from build123d import *

# Parameters (mm, degrees)
SKETCH1_R           = 3.25
SKETCH1_R_2         = 1.75
BOSS_EXTRUDE1_DEPTH = 10


with BuildPart() as part:
    # Sketch1 → Boss-Extrude1 (new body)
    with BuildSketch(Plane.XY):
        with BuildLine():
            Line((75.75, 8.25), (0, 8.25))
            ThreePointArc((0, 8.25), (-8.25, 0), (0, -8.25))
            Line((0, -8.25), (64.25, -8.25))
            Line((64.25, -8.25), (64.25, -19))
            ThreePointArc((64.25, -19), (70, -24.75), (75.75, -19))
            Line((75.75, -19), (75.75, 8.25))
        make_face()
        Circle(SKETCH1_R, mode=Mode.SUBTRACT)
        with Locations((70, -11)):
            Circle(SKETCH1_R_2, mode=Mode.SUBTRACT)
        with Locations((70, -19)):
            Circle(SKETCH1_R_2, mode=Mode.SUBTRACT)
    extrude(amount=BOSS_EXTRUDE1_DEPTH)


solid = part.part
The model under review builds one solid part; all positions refer to its coordinate system, in mm. A direction names the side the tool comes from. Give positions to 0.01 mm unless a question says otherwise; leave off trailing zeros. Write each loop counter-clockwise with the first axis right and the second up, starting at its lowest first coordinate (ties: lowest second). Pieces come first, ordered by that corner, then holes. Notation, with made-up numbers: M 4,81 L 56,81 A15 cw 56,106 Z; hole C -23.75,1 d3. An arc over 180 degrees is marked long. One line per question, with ' | ' between items. Start each with the question number.
Item 1: We need section D-D on y = -11. Write out the cut boundary in (x, z).
Item 2: For faces 4 (the flat face through (64.25, -14, 5)), 5 (the flat face through (75.75, -6, 5)), list the 3-axis set-ups (+Z, -Z, +X, -X, +Y, -Y) from which the entire face can be reached by the end or side of a thin tool; tool diameter is ignored.
Item 3: We need section B-B on x = 69. Write out the cut boundary in (y, z), plus the area to 3 significant figures.
Item 4: We need section A-A on y = 0. Write out the cut boundary in (x, z), plus the area to 3 significant figures.
Item 5: Draft analysis for pull direction Y (two halves, no side actions). For faces 1 (the flat face through (38, 8.25, 5)), 2 (the cylindrical face through (-2.579, -1.978, 4.93)), 3 (the flat face through (33, -1, 0)), state which applies: released by +Y, released by -Y, zero draft, split by the parting line, or undercut.
Item 6: Wall thickness on line 1 (Y direction, x = 70, z = 6.25); line 2 (Y direction, x = 0, z = 2.5); line 3 (Y direction, x = 71.5, z = 6.75): over which ranges is each line inside the solid? List them lowest first. Write a range as from..to.
Item 7: For pin 1 (1.5 mm diameter, centred on x = 36, z = 2.5, fed in from -Y); pin 2 (3 mm diameter, centred on y = -7, z = 7, fed in from -X); pin 3 (3 mm diameter, centred on x = 70, y = -11, fed in from +Z); pin 4 (3 mm diameter, centred on y = -13.5, z = 6, fed in from -X), all flat-tipped, find the tip position at first contact; note any pin that passes through.
Item 8: We need section C-C on z = 4.5. Write out the cut boundary in (x, y), plus the area to 3 significant figures.
Results found:
1) outline: M 64.25,0 L 68.25,0 L 68.25,10 L 64.25,10 Z; M 71.75,0 L 75.75,0 L 75.75,10 L 71.75,10 Z
2) face 4: +Z, -Z, -X, -Y | face 5: +Z, -Z, +X, +Y, -Y
3) outline: M -24.66,0 L -20.44,0 L -20.44,10 L -24.66,10 Z; M -17.56,0 L -12.44,0 L -12.44,10 L -17.56,10 Z; M -9.56,0 L 8.25,0 L 8.25,10 L -9.56,10 Z | area: 272 mm2
4) outline: M -8.25,0 L -3.25,0 L -3.25,10 L -8.25,10 Z; M 3.25,0 L 75.75,0 L 75.75,10 L 3.25,10 Z | area: 775 mm2
5) face 1: released by +Y | face 2: undercut | face 3: zero draft
6) line 1: y = -24.75..-20.75, -17.25..-12.75, -9.25..8.25 | line 2: y = -8.25..-3.25, 3.25..8.25 | line 3: y = -24.55..-19.9, -18.1..-11.9, -10.1..8.25
7) pin 1: stops at y = -8.25 | pin 2: stops at x = -6.15 | pin 3: passes through | pin 4: stops at x = 64.25
8) outline: M 0,-8.25 L 64.25,-8.25 L 64.25,-19 A5.75 ccw 75.75,-19 L 75.75,8.25 L 0,8.25 A8.25 ccw Z; hole C 0,0 d6.5; hole C 70,-19 d3.5; hole C 70,-11 d3.5 | area: 1,480 mm2
